from build123d import *

# Parameters (mm, degrees)
F0_R     = 9
F0_R_2   = 5
F1_DEPTH = 20
F2_R     = 1.6
F3_DEPTH = 7.1


with BuildPart() as f1:
    # F0 (on Top) → F1 (new body)
    with BuildSketch(Plane.XY):
        Circle(F0_R)
        Circle(F0_R_2, mode=Mode.SUBTRACT)
    extrude(amount=F1_DEPTH)

    # F2 (on Front) → F3 (cut)
    with BuildSketch(Plane.XZ):
        Polygon((-1.186389, 12.457307), (-3.144049, 9.957127), (-1.957661, 7.011654), (1.186389, 6.566359), (3.144049, 9.066539), (1.957661, 12.012013), align=None)
        with Locations((0, 9.511833)):
            Circle(F2_R, mode=Mode.SUBTRACT)
        with Locations((0, 9.511833)):
            Circle(F2_R)
    extrude(amount=-F3_DEPTH, mode=Mode.SUBTRACT)


solid = f1.part
Work out the finished part from the listing and answer in its coordinate system (mm). A direction names the side the tool comes from. Coordinates: 2 decimals unless noted, no trailing zeros. Write each loop counter-clockwise with the first axis right and the second up, starting at its lowest first coordinate (ties: lowest second). Pieces come first, ordered by that corner, then holes. Notation, with made-up numbers: M 1.5,69 L 28.5,69 A37 ccw 28.5,105 Z; hole C 79.25,33.5 d8. An arc over 180 degrees is marked long. Answer as CSV lines item,"result". Start each with the question number.
Item 1: Consider L1, parallel to Y at x = 0, z = 6.5; L2, parallel to Y at x = 0, z = 11.25; L3, parallel to X at y = -0.25, z = 12. Determine where each line is inside the solid, lowest interval first.
Item 2: Section A-A on y = 0 is taken. Write down the section's boundary in (x, z), and give its area (3 significant figures).
Item 3: Section D-D on z = 14.75 is taken. Write down the section's boundary in (x, y).
Item 4: A tool of negligible diameter and unlimited length cuts with its end or side. For faces 5 (the face through (0, 7.1, 10)), 6 (the face through (-1.08, -4.88, 9.86)), from which of +Z, -Z, +X, -X, +Y, -Y can it reach the whole face along a straight path? Write none if from no direction.
Item 5: Determine the mould class of faces 1 (the face through (-1.172, 8.923, 9.86)), 2 (the face through (4, -4, 20)), 3 (the face through (2.15, 5.83, 7.8)), 4 (the face through (-2.152, 5.828, 11.225)) for opening direction Y: released by +Y, released by -Y, zero draft, split by the parting line, or undercut.
Item 6: Flat-ended cylindrical pins translate along their axes: P1, Ø6, axis at y = 6, z = 13, coming from the +X side; P2, Ø3, axis at y = 5, z = 14.5, coming from the +X side; P3, Ø6, axis at y = -6.5, z = 6, coming from the -X side. Find the tip coordinate at first contact, or state that the pin passes through.
Item 7: Section C-C on y = -4.5 is taken. Write down the section's boundary in (x, z), and give its area (3 significant figures).
Item 8: Section B-B on x = 0 is taken. Write down the section's boundary in (y, z).
Checks:
1,L1,"y = -9 to -5, 5 to 9"
1,L2,"y = -9 to -5, 7.1 to 9"
1,L3,"x = -9 to -4.99, 4.99 to 9"
2,outline,"M -9,0 L -5,0 L -5,20 L -9,20 Z; M 5,0 L 9,0 L 9,20 L 5,20 Z"
2,area,"160 mm²"
3,outline,"C 0,0 d18; hole C 0,0 d10"
4,face 5,"none"
4,face 6,"+Z, -Z"
5,face 1,"split by the parting line"
5,face 2,"zero draft"
5,face 3,"undercut"
5,face 4,"undercut"
6,P1,"stops at x = 8.49"
6,P2,"stops at x = 8.29"
6,P3,"stops at x = -8.29"
7,outline,"M -7.79,0 L -2.18,0 L -2.18,20 L -7.79,20 Z; M 2.18,0 L 7.79,0 L 7.79,20 L 2.18,20 Z"
7,area,"225 mm²"
8,outline,"M -9,0 L -5,0 L -5,20 L -9,20 Z; M 5,0 L 9,0 L 9,20 L 5,20 L 5,12.29 L 7.1,12.29 L 7.1,6.73 L 5,6.73 Z"
